from build123d import *

# Parameters (mm, degrees)
SKETCH_1_W                       = 12
SKETCH_1_H                       = 61.85
EXTRUDE_1_DEPTH                  = 6
SKETCH_2_W                       = 24
SKETCH_2_H                       = 10.13
EXTRUDE_2_DEPTH                  = 4
SKETCH_3_R                       = 1.5
CUT_EXTRUDE_1_DEPTH              = 4
FILLET_1_R                       = 2
PATTERN_CIRCULAR_1_COUNT         = 3
FILLET_1_OF_PATTERN_CIRCULAR_1_R = 2
FILLET_2_R                       = 10


with BuildPart() as part:
    # Sketch 1 → Extrude 1 (new body)
    with BuildSketch(Plane(origin=(0, 0, 0), x_dir=(1, 0, 0), z_dir=(0, 1, 0))):
        with Locations((0, 30.925)):
            Rectangle(SKETCH_1_W, SKETCH_1_H)
    extrude_1 = extrude(amount=EXTRUDE_1_DEPTH)

    # Sketch 2 → Extrude 2 (add)
    with BuildSketch(Plane(origin=(0, 0, -61.85), x_dir=(-1, 0, 0), z_dir=(0, 0, -1))):
        with Locations((0, 5.065)):
            Rectangle(SKETCH_2_W, SKETCH_2_H)
    extrude_2 = extrude(amount=-EXTRUDE_2_DEPTH)

    # Sketch 3 → Cut-Extrude 1 (cut)
    with BuildSketch(Plane.XY.offset(-57.85)):
        with Locations((-9, 4)):
            Circle(SKETCH_3_R)
        with Locations((9, 4)):
            Circle(SKETCH_3_R)
    cut_extrude_1 = extrude(amount=-CUT_EXTRUDE_1_DEPTH, mode=Mode.SUBTRACT)

    # Fillet 1
    fillet_1_edges = [part.edges().sort_by_distance(p)[0] for p in [
        (0, 6, -57.85),
    ]]
    fillet(fillet_1_edges, radius=FILLET_1_R)

    # Pattern Circular 1: Extrude 1, Extrude 2, Cut-Extrude 1 ×3 about axis
    pattern_circular_1_axis = Axis((0, 0, 0), (0, 1, 0))
    add([extrude_1.rotate(pattern_circular_1_axis, i * 360 / PATTERN_CIRCULAR_1_COUNT) for i in range(1, PATTERN_CIRCULAR_1_COUNT)])
    add([extrude_2.rotate(pattern_circular_1_axis, i * 360 / PATTERN_CIRCULAR_1_COUNT) for i in range(1, PATTERN_CIRCULAR_1_COUNT)])
    add([cut_extrude_1.rotate(pattern_circular_1_axis, i * 360 / PATTERN_CIRCULAR_1_COUNT) for i in range(1, PATTERN_CIRCULAR_1_COUNT)], mode=Mode.SUBTRACT)

    # Fillet 1 of Pattern Circular 1
    fillet_1_of_pattern_circular_1_edges = [part.edges().sort_by_distance(p)[0] for p in [
        (-50.099569609, 6, 28.925),
        (50.099569609, 6, 28.925),
    ]]
    fillet(fillet_1_of_pattern_circular_1_edges, radius=FILLET_1_OF_PATTERN_CIRCULAR_1_R)

    # Fillet 2
    fillet_2_edges = [part.edges().sort_by_distance(p)[0] for p in [
        (6, 3, -3.464101615),
        (-6, 3, -3.464101615),
        (0, 3, 6.92820323),
    ]]
    fillet(fillet_2_edges, radius=FILLET_2_R)


solid = part.part
Geometry: final body of the model. Coordinates: model frame, mm. A direction names the side the tool comes from. Round coordinates to 2 decimals unless told otherwise and drop trailing zeros. Order: outer loops, then holes, each group sorted by start corner. A loop starts at its lowest first (then second) coordinate and runs counter-clockwise, first axis right, second up. Notation, with made-up numbers: (-36.75, 24) -> (15.25, 24) arc R24 ccw to (15.25, 46) -> close; hole circle Ø4 at (68.5, 55.25). An arc over 180 degrees is marked (long way). Put each result on its own line as item: value. Start each with the question number.
Q1. Pull-direction query (X, two-part tool) for faces 1 (the cylindrical face through (-49.564, 6.601, 28.713)), 2 (the cylindrical face through (-7.303, 3.042, -4.301)), 3 (the cylindrical face through (7.38, 2.96, -4.17)); classes: +X half, -X half, draft (parallel to the pull), parting line (faces both ways), or undercut.
Q2. Line query: probe 1 along Y at (x, z) = (9, -59.85); probe 2 along Y at (x, z) = (-3.5, -18.5); probe 3 along X at (y, z) = (1.75, -23.5). Output: solid intervals per line, ascending.
Q3. Section D-D on z = -33.5. Return the cut outline in (x, y), and give its area (3 significant figures).
Q4. Section C-C on y = 4. Give the number of separate pieces and of enclosed holes in the cut face, and give its area (3 significant figures).
Q5. First-contact query: pin 1 (5 mm diameter, centred on x = 5, y = 7.5, fed in from +Z); pin 2 (6 mm diameter, centred on x = 8.5, z = -32.5, fed in from +Y); pin 3 (5 mm diameter, centred on y = 8, z = -35, fed in from -X); pin 4 (5 mm diameter, centred on x = 9, y = 4, fed in from -Z). Flat tips, straight axial feed; report the tip coordinate or a pass-through.
Q6. Section B-B on z = 12. Return the cut outline in (x, y).
Q7. Section A-A on x = -9. Return the cut outline in (y, z), and give its area (3 significant figures).
Q8. Reachability of faces 4 (the flat face through (0, 9, -57.85)), 5 (the flat face through (-12, 5, -60)), 6 (the cylindrical face through (49.648, 6.601, 28.567)), 7 (the flat face through (45.856, 4.994, 40.331)) from +Z, -Z, +X, -X, +Y, -Y: full face, straight path, thin tool, end or side. Return the list, or none.
Ans:
1. face 1: undercut
1. face 2: -X half
1. face 3: +X half
2. probe 1: y = 0 to 2.5, 5.5 to 10.13
2. probe 2: y = 0 to 6
2. probe 3: x = -6 to 6
3. outline: (-6, 0) -> (6, 0) -> (6, 6) -> (-6, 6) -> close
3. area: 72.0 mm2
4. separate pieces: 7
4. enclosed holes: 0
4. area: 2,250 mm2
5. pin 1: stops at z = 10.97
5. pin 2: stops at y = 6
5. pin 3: stops at x = -6
5. pin 4: stops at z = -61.85
6. outline: (-32.78, 0) -> (-8.78, 0) -> (-8.78, 6) -> (-32.78, 6) -> close; (8.78, 0) -> (32.78, 0) -> (32.78, 6) -> (8.78, 6) -> close
7. outline: (0, -61.85) -> (2.5, -61.85) -> (2.5, -57.85) -> (0, -57.85) -> close; (0, -2.1) -> (6, -2.1) -> (6, 12.12) -> (0, 12.12) -> close; (5.5, -61.85) -> (10.13, -61.85) -> (10.13, -57.85) -> (5.5, -57.85) -> close
7. area: 114 mm2
8. face 4: +Y
8. face 5: -Z, -X, +Y, -Y
8. face 6: -Z, +Y
8. face 7: +Z, +Y, -Y
